Part model, mm, in its own coordinate system. A direction names the side the tool comes from. Round coordinates to 2 decimals unless told otherwise and drop trailing zeros. Write each loop counter-clockwise with the first axis right and the second up, starting at its lowest first coordinate (ties: lowest second). Pieces come first, ordered by that corner, then holes.
1) Saw through at C-C on x = -8. Write the cut outline in (y, z).
2) Which spindle directions (+Z, -Z, +X, -X, +Y, -Y) get a long thin tool onto all of the face, cutting with end or side? Do faces 4 (the flat face through (29.438, -12.325, 7.276)), 5 (the cylindrical face through (8.859, -23.496, 60.199)). Say none if no direction does.
3) Saw through at A-A on z = 3.5. Write the cut outline in (x, y), and give its area (3 significant figures).
4) Flat gauge pins, fed straight in: pin 1 (12 mm diameter, centred on x = 6.5, z = -22.5, fed in from +Y); pin 2 (5 mm diameter, centred on x = 41.5, y = -5.5, fed in from +Z); pin 3 (10 mm diameter, centred on y = -9.5, z = 28.5, fed in from -X); pin 4 (1.5 mm diameter, centred on x = -40, y = -21, fed in from +Z). Where does each tip first touch, or does it go through?
5) Pull direction X, two halves, no side cores. Call faces 1 (the flat face through (-36.978, -9.86, 37.855)), 2 (the flat face through (4, -25, 22)), 3 (the flat face through (1.656, -12.325, -9.75)): +X half, -X half, draft (parallel to the pull), parting line (faces both ways), or undercut.
6) Saw through at B-B on y = -13.5. Write the cut outline in (x, z), and give its area (3 significant figures).
7) Drill centre lines: L1, parallel to X at y = -12.5, z = 28; L2, parallel to Z at x = -16.5, y = -3.75; L3, parallel to Z at x = -13, y = -1.5. Where is each one in solid material? Low to high.
8) Saw through at D-D on z = -18.5. Write the cut outline in (x, y), and give its area (3 significant figures).
```python
from build123d import *

# Parameters (mm, degrees)
F1_DEPTH = 25
F2_R     = 5


with BuildPart() as f1:
    # F0 (on Front) → F1 (new body)
    with BuildSketch(Plane.XZ):
        Polygon((-58.095872, 13.411373), (-16.461365, -33.184543), (20.287085, 14.35025), (38.849397, 0), (67.183668, 36.650898), (34.879841, 61.624512), (-16.44367, 61.624512), align=None)
    extrude(amount=F1_DEPTH)

    # F2
    f2_edges = [f1.edges().sort_by_distance(p)[0] for p in [
        (51.031754, -25, 49.137705),
        (9.218086, -25, 61.624512),
        (-37.269771, -25, 37.517942),
    ]]
    fillet(f2_edges, radius=F2_R)


solid = f1.part
```
Completed:
1. outline: (-25, -22.24) - (0, -22.24) - (0, 61.62) - (-20, 61.62) arc R5 ccw to (-25, 56.62) - close
2. face 4: -Z, +Y, -Y
2. face 5: +Z, +X, -X, -Y
3. outline: (-49.24, -25) - (11.9, -25) - (11.9, 0) - (-49.24, 0) - close; (34.32, -25) - (41.56, -25) - (41.56, 0) - (34.32, 0) - close
3. area: 1,710 mm2
4. pin 1: passes through
4. pin 2: stops at z = 58.44
4. pin 3: stops at x = -49.38
4. pin 4: stops at z = 35.1
5. face 1: -X half
5. face 2: draft
5. face 3: undercut
6. outline: (-58.1, 13.41) - (-16.46, -33.18) - (20.29, 14.35) - (38.85, 0) - (67.18, 36.65) - (34.88, 61.62) - (-16.44, 61.62) - close
6. area: 6,420 mm2
7. L1: x = -45.49 to 60.5
7. L2: z = -33.14 to 61.56
7. L3: z = -28.71 to 61.62
8. outline: (-29.58, -25) - (-5.11, -25) - (-5.11, 0) - (-29.58, 0) - close
8. area: 612 mm2
